Solid Edge part; units mm, degrees
sketch "Sketch1" plane through (0, 0, 0) normal (0, -1, 0) x (1, 0, 0)
  line L0 (-5.3694, 18.9) -> (-19.0694, -4.8291)
  arc A0 (-13.7, -14.1291) -> (-19.0694, -4.8291) centre (-13.7, -7.9291) cw
  line L1 (-13.7, -14.1291) -> (13.7, -14.1291)
  arc A1 (19.0694, -4.8291) -> (13.7, -14.1291) centre (13.7, -7.9291) cw
  line L2 (5.3694, 18.9) -> (19.0694, -4.8291)
  arc A2 (-5.3694, 18.9) -> (5.3694, 18.9) centre (0, 15.8) cw
  dimension "D1" = 5.3694
extrude "Protrusion1" add sketch "Sketch1" against normal blind 14
sketch "Sketch2" plane through (0, 0, 0) normal (0, -1, 0) x (1, 0, 0)
  circle A0 centre (-13.7, -7.9291) radius 2.2
  circle A1 centre (13.7, -7.9291) radius 2.2
  circle A2 centre (0, 15.8) radius 2.2
extrude "Cutout1" cut sketch "Sketch2" against normal blind 457.8755
sketch "Sketch3" plane through (0, 0, 0) normal (0, -1, 0) x (1, 0, 0)
  circle A0 centre (0, 0) radius 7.7
extrude "Cutout2" cut sketch "Sketch3" against normal blind 434.4917
sketch "Sketch4" plane through (0, 0, 3.9355) normal (0, -1, 0) x (-0.5, 0, 0.8660254)
  line L0 (-23.325, -5.9323) -> (-23.325, -18.9323)
  line L1 (-23.325, -18.9323) -> (16.475, -18.9323)
  line L2 (16.475, -18.9323) -> (16.475, -5.9323)
  line L3 (12.7755, -8.7037) -> (16.475, -5.9323)
  line L4 (-20.9306, -8.7037) -> (12.7755, -8.7037)
  line L5 (-20.9306, -5.9323) -> (-20.9306, -8.7037)
  line L6 (-23.325, -5.9323) -> (-20.9306, -5.9323)
  dimension "D1" = 23.325
extrude "Protrusion2" add sketch "Sketch4" against normal up to vertex (14 mm away)
sketch "Sketch5" plane through (18.1083, 8, 10.4355) normal (0.8660254, 0, 0.5) x (-0.5, 0, 0.8660254)
  line L0 (-19.9, 8) -> (19.9, 8)
  line L1 (19.9, -6) -> (19.9, 8)
  line L2 (-19.9, -6) -> (19.9, -6)
  line L3 (-19.9, -6) -> (-19.9, 8)
extrude "ExtrudedProtrusion_14" add sketch "Sketch5" along normal blind 4
sketch "Sketch6" plane through (11.8615, 14, 7.7701) normal (0, 1, 0) x (-0.8660254, 0, -0.5)
  circle A0 centre (-2.5426, -0.8152) radius 2.2
extrude "ExtrudedCutout_23" cut sketch "Sketch6" against normal blind 166.5817
sketch "Sketch7" plane through (11.8615, 14, 7.7701) normal (0, 1, 0) x (-0.8660254, 0, -0.5)
  circle A0 centre (40.6865, -0.8152) radius 2.2
  line L0 (40.6865, 5.6848) -> (31.1282, 5.6848)
  line L1 (31.1282, 5.6848) -> (31.1282, 3.8832)
  line L2 (31.1282, 3.8832) -> (34.2429, 1.8592)
  line L3 (34.2429, 1.8592) -> (34.2429, -2.6486)
  line L4 (31.1282, -7.3152) -> (34.2429, -2.6486)
  line L5 (40.6865, -7.3152) -> (31.1282, -7.3152)
  arc A1 (40.6865, -7.3152) -> (40.6865, 5.6848) centre (40.6865, -0.8152) ccw
extrude "Protrusion3" add sketch "Sketch7" against normal up to vertex (14 mm away)
sketch "Sketch8" plane through (11.8615, 14, 7.7701) normal (0, 1, 0) x (-0.8660254, 0, -0.5)
  line L0 (-10.7426, -0.8152) -> (-10.7426, -20.7152)
  line L1 (-10.7426, -20.7152) -> (6.2574, -20.7152)
  arc A0 (1.1563, -18.0392) -> (6.2574, -20.7152) centre (6.2574, -14.5152) ccw
  line L2 (1.1563, -18.0392) -> (-10.7426, -0.8152)
extrude "Cutout3" cut sketch "Sketch8" against normal blind 85.4791
sketch "Sketch9" plane through (6.8865, 14, 7.7701) normal (0, 1, 0) x (-0.8660254, 0, -0.5)
  line L0 (-15.0511, 16.5973) -> (-15.0511, -3.3027)
  line L1 (-3.1522, 13.9213) -> (-15.0511, -3.3027)
  arc A0 (1.9489, 16.5973) -> (-3.1522, 13.9213) centre (1.9489, 10.3973) ccw
  line L2 (1.9489, 16.5973) -> (-15.0511, 16.5973)
extrude "ExtrudedCutout_27" cut sketch "Sketch9" against normal blind 118.3722
fillet "Round_1" radius 6.6 1 edges at (21.5724, 7, 12.4355)
The model under review builds one solid part; all positions refer to its coordinate system, in mm. A direction names the side the tool comes from. Round coordinates to 2 decimals unless told otherwise and drop trailing zeros. Loops run counter-clockwise (first coordinate to the right, second up) from the corner with the lowest first, then second, coordinate; pieces in that order, holes last. Notation, with made-up numbers: (86.25, 67.25) -> (101.25, 67.25) arc R19 ccw to (101.25, 101.25) -> close; hole circle Ø11 at (-28, -38). An arc over 180 degrees is marked (long way). Answer in a Markdown table with one row per item.
1) For pin 1 Ø5 at (x, y) = (12.5, 12) entering from +Z; pin 2 Ø8 at (x, y) = (-18, 4) entering from -Z; pin 3 Ø1 at (x, y) = (4, 4.5) entering from +Z; pin 4 Ø4 at (x, z) = (-22.97, -13.28) entering from +Y, all flat-tipped, find the tip position at first contact; note any pin that passes through.
Taken from the geometry:
| item | result |
|---|---|
| pin 1 | stops at z = 17.92 |
| pin 2 | stops at z = -19.71 |
| pin 3 | stops at z = 21 |
| pin 4 | passes through |
2) Consider section A-A, the plane x = 0. Write out the cut boundary in (y, z), plus the area to 3 significant figures.
Taken from the geometry:
| item | result |
|---|---|
| outline | (0, -14.13) -> (14, -14.13) -> (14, -7.7) -> (0, -7.7) -> close; (0, 7.7) -> (14, 7.7) -> (14, 13.6) -> (0, 13.6) -> close; (0, 18) -> (14, 18) -> (14, 22) -> (0, 22) -> close |
| area | 229 mm² |
3) Wall thickness on line 1 along Z through (x, y) = (0, 5.5); line 2 along X through (y, z) = (3.5, -4); line 3 along Z through (x, y) = (13.7, 11.25): over which ranges is each line inside the solid? List them lowest first.
Taken from the geometry:
| item | result |
|---|---|
| line 1 | z = -14.13 to -7.7, 7.7 to 13.6, 18 to 22 |
| line 2 | x = -19.89 to -6.58, 6.58 to 20.24 |
| line 3 | z = -14.13 to -10.13, -5.73 to 6.27, 10.4 to 16.17 |
4) Tool access review of faces 1 (the flat face through (1, 7, -14.129)), 2 (the flat face through (-22.136, 7.098, -5.294)): name each direction out of +Z, -Z, +X, -X, +Y, -Y from which nothing blocks a thin tool from reaching the whole face with its end or side.
Taken from the geometry:
| item | result |
|---|---|
| face 1 | -Z, +X, +Y, -Y |
| face 2 | +Z, -X, +Y, -Y |
5) Consider section B-B, the plane z = -3.5. Write out the cut boundary in (x, y), plus the area to 3 significant figures.
Taken from the geometry:
| item | result |
|---|---|
| outline | (-19.03, 0) -> (-6.86, 0) -> (-6.86, 14) -> (-19.03, 14) -> close; (6.86, 0) -> (20.28, 0) -> (20.28, 14) -> (6.86, 14) -> close |
| area | 358 mm² |
6) Consider section C-C, the plane x = -13.7. Write out the cut boundary in (y, z).
Taken from the geometry:
| item | result |
|---|---|
| outline | (0, -15.43) -> (14, -15.43) -> (14, -10.13) -> (0, -10.13) -> close; (0, -5.73) -> (14, -5.73) -> (14, 4.47) -> (0, 4.47) -> close |
7) Draft analysis for pull direction X (two halves, no side actions). For faces 3 (the flat face through (2, 0, -8)), 4 (the cylindrical face through (20.369, 6.902, 11.676)), 5 (the cylindrical face through (-11.668, 6.902, -8.772)), 6 (the cylindrical face through (-1.669, 6.902, -7.517)), state which applies: pulls with the +X half, pulls with the -X half, needs draft (parallel to the pull), parting line crosses it, or undercut.
Taken from the geometry:
| item | result |
|---|---|
| face 3 | needs draft |
| face 4 | pulls with the +X half |
| face 5 | undercut |
| face 6 | undercut |
